Could you check a few things on this model? Use its own coordinates, in mm. A direction names the side the tool comes from. Round coordinates to 2 decimals unless told otherwise and drop trailing zeros. Loops run counter-clockwise (first coordinate to the right, second up) from the corner with the lowest first, then second, coordinate; pieces in that order, holes last. Notation, with made-up numbers: (25, 61) -> (54, 61) arc R27 cw to (54, 99) -> close; hole circle Ø6 at (71.25, 53). An arc over 180 degrees is marked (long way). Put each result on its own line as item: value. Start each with the question number.
1. I'm going to push flat-ended pins straight in: P1, Ø6, axis at x = -1, y = 6.5, coming from the +Z side; P2, Ø4, axis at y = 17.5, z = 2, coming from the -X side; P3, Ø1.5, axis at y = 3.5, z = -0.5, coming from the +X side; P4, Ø5, axis at y = 14, z = -1, coming from the +X side. Where does each tip first touch, or does it pass through?
2. I need wall thicknesses on line 1 (X direction, y = 29, z = 3); line 2 (X direction, y = 23, z = 1.75); line 3 (Z direction, x = -2, y = 9.5). Which ranges of each line are inside material? Lowest first, please. Write a range as [from, to].
3. Imagine slicing it at B-B, the plane x = -7. Please give me the cut outline in (y, z).
4. Imagine slicing it at A-A, the plane y = 23. Please give me the cut outline in (x, z).
5. If we mould it in two halves opening along X, with no side actions, what happens to faces 1 (the cylindrical face through (0, -3.5, 0.1)), 2 (the cylindrical face through (-9.88, 37.82, 3.93)), 3 (the cylindrical face through (0.019, 2.273, -2.726)), 4 (the flat face through (10.014, 38.407, 0.035))? For each: pulls with the +X half, pulls with the -X half, needs draft (parallel to the pull), parting line crosses it, or undercut.
6. Which directions (+Z, -Z, +X, -X, +Y, -Y) give clear straight access to the entire face, cutting with the end or side of a thin tool? Please do faces 5 (the cylindrical face through (-1.421, 10.322, 0.014)), 6 (the cylindrical face through (-13.671, 36.584, -1.331)), 7 (the cylindrical face through (0.019, 2.273, 2.774)).
```python
from build123d import *

# Parameters (mm, degrees)
F1_DEPTH      = 4.5
F1_DEPTH_BACK = 4.5
F3_DEPTH      = 1
F3_DEPTH_BACK = 1
F4_R          = 3.475
F5_DEPTH      = 8
F6_R          = 2
F8_R          = 2


with BuildPart() as f1:
    # F0 (on Top) → F1 (new body, two sides)
    with BuildSketch(Plane.XY) as f1_sk:
        with BuildLine():
            Line((-10.9997768011, 38.1843295809), (-1.9510017572, -1.9396118641))
            ThreePointArc((-1.9510017572, -1.9396118641), (0, -3.499620792), (1.9510017572, -1.9396118641))
            Line((1.9510017572, -1.9396118641), (10.9997768011, 38.1843295809))
            Line((10.9997768011, 38.1843295809), (9, 38.6353204298))
            Line((9, 38.6353204298), (0.9755008786, 3.0532077891))
            ThreePointArc((0.9755008786, 3.0532077891), (0, 2.2732033252), (-0.9755008786, 3.0532077891))
            Line((-0.9755008786, 3.0532077891), (-9, 38.6353204298))
            Line((-9, 38.6353204298), (-10.9997768011, 38.1843295809))
        make_face()
    extrude(amount=F1_DEPTH)
    extrude(f1_sk.sketch, amount=-F1_DEPTH_BACK)

    # F2 (on Top) → F3 (join, two sides)
    with BuildSketch(Plane.XY) as f3_sk:
        with BuildLine():
            ThreePointArc((4.067072408, 12.170038485), (0.0224234698, 10.1095648017), (-4.0222254685, 12.170038485))
            Line((-4.0222254685, 12.170038485), (-1.7974023818, -0.8990558693))
            Line((-1.7974023818, -0.8990558693), (1.8422493213, -0.8990558693))
            Line((1.8422493213, -0.8990558693), (4.067072408, 12.170038485))
        make_face()
    extrude(amount=F3_DEPTH)
    extrude(f3_sk.sketch, amount=-F3_DEPTH_BACK)

    # F4 (on face) → F5 (join)
    with BuildSketch(Plane(origin=(2.2728291349, -0.5125697729, 0), x_dir=(0.219995536, 0.9755008786, 0), z_dir=(0.9755008786, -0.219995536, 0))):
        with Locations((35.4849845171, 0)):
            Circle(F4_R)
    extrude(amount=F5_DEPTH)

    # F6
    f6_edges = [f1.edges().sort_by_distance(p)[0] for p in [
        (17.11889, 28.953234, 0),
    ]]
    fillet(f6_edges, radius=F6_R)

    # F7: F1 across plane


with BuildPart() as f1_1:
    add(f1.part)
    add(f1.part.mirror(Plane.YZ))

    # F8
    f8_edges = [f1_1.edges().sort_by_distance(p)[0] for p in [
        (9.999888, 38.409825, 4.5),
        (9.999888, 38.409825, -4.5),
        (-9.999888, 38.409825, -4.5),
        (-9.999888, 38.409825, 4.5),
    ]]
    fillet(f8_edges, radius=F8_R)


solid = f1_1.part
```
Entries:
1. P1: z = 4.5
1. P2: x = -6.79
1. P3: x = 3.35
1. P4: x = 6.11
2. line 1: [-8.93, -6.83], [6.83, 8.93]
2. line 2: [-7.58, -5.47], [5.47, 7.58]
2. line 3: [-1, 1]
3. outline: (20.45, -4.5) -> (29.77, -4.5) -> (29.77, 4.5) -> (20.45, 4.5) -> close
4. outline: (-7.58, -4.5) -> (-5.47, -4.5) -> (-5.47, 4.5) -> (-7.58, 4.5) -> close; (5.47, -4.5) -> (7.58, -4.5) -> (7.58, 4.5) -> (5.47, 4.5) -> close
5. face 1: parting line crosses it
5. face 2: pulls with the -X half
5. face 3: undercut
5. face 4: pulls with the +X half
6. face 5: +Z, -Z, +Y
6. face 6: none
6. face 7: +Z, +Y
